CAD build for the part. Positions are in the model's coordinates, mm. A direction names the side the tool comes from. Coordinates: 2 decimals unless noted, no trailing zeros. Order: outer loops, then holes, each group sorted by start corner. A loop starts at its lowest first (then second) coordinate and runs counter-clockwise, first axis right, second up. Notation, with made-up numbers: M 84.25,70 L 104.25,70 A32 ccw 104.25,109 Z; hole C -13,41.25 d7. An arc over 180 degrees is marked long. One line per item, written item: value.
from build123d import *

# Parameters (mm, degrees)
SKETCH1_W           = 138
SKETCH1_H           = 95
BOSS_EXTRUDE1_DEPTH = 15
SKETCH2_W           = 128
SKETCH2_H           = 86
CUT_EXTRUDE1_DEPTH  = 7
SNAP_START          = 64.5
SNAP_HOOK2_DEPTH    = 2
SNAP_HOOK2_2_DEPTH  = 2
FILLET1_R           = 1
FILLET2_R           = 0.5
BOSS_EXTRUDE2_DEPTH = 2
FILLET3_R           = 0.5
FILLET4_R           = 0.5
FILLET7_R           = 0.1


with BuildPart() as part:
    # Sketch1 → Boss-Extrude1 (new body)
    with BuildSketch(Plane(origin=(0, 0, 0), x_dir=(1, 0, 0), z_dir=(0, 1, 0))):
        Rectangle(SKETCH1_W, SKETCH1_H)
    extrude(amount=BOSS_EXTRUDE1_DEPTH)

    # Sketch2 → Cut-Extrude1 (cut)
    with BuildSketch(Plane(origin=(0, 15, 0), x_dir=(1, 0, 0), z_dir=(0, 1, 0))):
        Rectangle(SKETCH2_W, SKETCH2_H)
    extrude(amount=-CUT_EXTRUDE1_DEPTH, mode=Mode.SUBTRACT)



with BuildPart() as body_2:
    # Snap Hook2: read off the stored shape, not the designer's step
    # Snap Hook2 outline → Snap Hook2 (new body)
    with BuildSketch(Plane.YZ.offset(SNAP_START)):
        Polygon((21, -2), (21, 2), (18, 2.157223338), (18, -2.157223338), align=None)
    snap_hook2 = extrude(amount=SNAP_HOOK2_DEPTH)


with BuildPart() as part_1:
    add(part.part)

    add(body_2.part)  # Snap Hook2 2 merges body 2
    # Snap Hook2 2 outline → Snap Hook2 2 (add)
    with BuildSketch(Plane.YZ.offset(SNAP_START)):
        Polygon((18, -2.157223338), (18, 2.157223338), (15, 2.314446676), (15, -2.314446676), align=None)
    snap_hook2_2 = extrude(amount=SNAP_HOOK2_2_DEPTH)

    # Snap Hook2 3: loft between two sections, ruled curve by curve
    snap_hook2_3_from = [
        Edge.make_line((66.5, 21, -2), (66.5, 21, 2)),
        Edge.make_line((66.5, 18, 2.157223338), (66.5, 18, -2.157223338)),
        Edge.make_line((66.5, 18, 2.157223338), (66.5, 21, 2)),
        Edge.make_line((66.5, 18, -2.157223338), (66.5, 21, -2)),
    ]
    snap_hook2_3_to = [
        Edge.make_line((68.5, 19, -2.104815559), (68.5, 19, 2.104815559)),
        Edge.make_line((68.5, 18, 2.157223338), (68.5, 18, -2.157223338)),
        Edge.make_line((68.5, 18, 2.157223338), (68.5, 19, 2.104815559)),
        Edge.make_line((68.5, 18, -2.157223338), (68.5, 19, -2.104815559)),
    ]
    snap_hook2_3 = Solid(Shell([*[Face.make_surface_from_curves(snap_hook2_3_from[k], snap_hook2_3_to[k]) for k in range(4)], Face(Wire(snap_hook2_3_from)), Face(Wire(snap_hook2_3_to))]))
    add(snap_hook2_3)

    # Fillet1
    fillet1_edges = [part_1.edges().sort_by_distance(p)[0] for p in [
        (64, 11.5, -43),
        (64, 11.5, 43),
        (-64, 11.5, 43),
        (-64, 11.5, -43),
        (-69, 7.5, -47.5),
        (69, 7.5, -47.5),
        (69, 7.5, 47.5),
        (-69, 7.5, 47.5),
    ]]
    fillet(fillet1_edges, radius=FILLET1_R)

    # Mirror1: Snap Hook2, Snap Hook2 2, Snap Hook2 3 across plane
    add(snap_hook2.mirror(Plane(origin=(0, 0, 0), x_dir=(0, 0, 1), z_dir=(1, 0, 0))))
    add(snap_hook2_2.mirror(Plane(origin=(0, 0, 0), x_dir=(0, 0, 1), z_dir=(1, 0, 0))))
    add(snap_hook2_3.mirror(Plane(origin=(0, 0, 0), x_dir=(0, 0, 1), z_dir=(1, 0, 0))))

    # Fillet2
    fillet2_edges = [part_1.edges().sort_by_distance(p)[0] for p in [
        (66.5, 15, 0),
        (64.5, 15, 0),
        (-66.5, 15, 0),
        (-64.5, 15, 0),
    ]]
    fillet(fillet2_edges, radius=FILLET2_R - 0.0001)  # a hair under: the kernel refuses the full size

    # Sketch5 → Boss-Extrude2 (add)
    with BuildSketch(Plane.ZY.offset(68.5)):
        Polygon((-2.104815559, 19), (2.104815559, 19), (2.189499682, 17.384130663), (-2.189499682, 17.384130663), align=None)
    extrude(amount=BOSS_EXTRUDE2_DEPTH)

    # Cut-Sweep1: sweep along a curve in space
    with BuildLine() as cut_sweep1_path:
        Line((-70.5, 17.384130663, -2.189499682), (-70.5, 17.384130663, 2.189499682))
    # Sketch6 → Cut-Sweep1 (sweep, cut)
    with BuildSketch(Plane(origin=(0, 0.162048562, -3.09207076), x_dir=(-1, 0, 0), z_dir=(0, 0.052335956242943814, -0.998629534754574))):
        Polygon((68.5, 17.862431279), (69.245478091, 17.245716756), (68.5, 17.245716756), align=None)
    sweep(path=cut_sweep1_path.line, mode=Mode.SUBTRACT)

    # Cut-Sweep2: sweep along a curve in space
    with BuildLine() as cut_sweep2_path:
        Line((-70.5, 17.384130663, -2.189499682), (-70.5, 17.384130663, 2.189499682))
    # Sketch7 → Cut-Sweep2 (sweep, cut)
    with BuildSketch(Plane(origin=(0, 0.162048562, -3.09207076), x_dir=(-1, 0, 0), z_dir=(0, 0.052335956242943814, -0.998629534754574))):
        Polygon((68.5, 18.863803625), (69.5, 17.245716756), (70.5, 17.245716756), (70.5, 18.863803625), align=None)
    sweep(path=cut_sweep2_path.line, mode=Mode.SUBTRACT)

    # Fillet3
    # the kernel refuses this fillet: 0.5 mm, written as the material it adds along each edge
    with BuildSketch(Plane(origin=(-68.5, 18, 2.606776404), x_dir=(1, 0, 0), z_dir=(0, 0, -1))) as fillet3_piece_1_section:
        with BuildLine():
            CenterArc((FILLET3_R * 0.359642452732, FILLET3_R), FILLET3_R, 230.43852258, 39.56147742)
            Line((-FILLET3_R * 0.277263341593, FILLET3_R * 0.22905836203), (0, 0))
            Line((0, 0), (FILLET3_R * 0.359642452732, 0))
        make_face()
    fillet3_piece_1 = extrude(amount=5.213552808, mode=Mode.PRIVATE)
    fillet3_piece_1 = split(fillet3_piece_1, bisect_by=Plane(origin=(-68.5, 17.976504454, 2.158454687), z_dir=(0, -0.052335956242943654, -0.9986295347545739)), keep=Keep.TOP, mode=Mode.PRIVATE)
    fillet3_piece_1 = split(fillet3_piece_1, bisect_by=Plane(origin=(-68.5, 18.248986786, -2.144174493), z_dir=(0, -0.05233595624294393, 0.9986295347545739)), keep=Keep.TOP, mode=Mode.PRIVATE)
    add(fillet3_piece_1)
    # the kernel refuses this fillet: 0.5 mm, written as the material it takes off along each edge
    with BuildSketch(Plane(origin=(-68.5, 19, -2.249978478), x_dir=(0.7071067811865781, 0.7071067811865169, 0), z_dir=(0, 0, 1))) as fillet3_2_piece_1:
        with BuildLine():
            CenterArc((FILLET3_R * 0.11613033532, -FILLET3_R), FILLET3_R, 90, 13.248212602)
            Line((-FILLET3_R * 0.11303968997, -FILLET3_R * 0.0266135918822), (0, 0))
            Line((0, 0), (FILLET3_R * 0.11613033532, 0))
        make_face()
    extrude(amount=4.499956956, mode=Mode.SUBTRACT)

    # Fillet4
    # the kernel refuses this fillet: 0.5 mm, written as the material it takes off along each edge
    with BuildSketch(Plane(origin=(-69.5, 17.384130663, -3.553874189), x_dir=(0.5262404509675064, 0.8503358088223238, 0), z_dir=(0, 0, 1))) as fillet4_piece_1:
        with BuildLine():
            CenterArc((0.545749803, -0.5), FILLET4_R, 90, 55.448844763)
            Line((0.133939724, -0.216429093), (0.125703523, -0.210757675))
            ThreePointArc((0.125703523, -0.210757675), (0.058466504, -0.113476951), (-0.008503358, -0.005262405))
            Line((-0.008503358, -0.005262405), (0, 0.01))
            Line((0, 0.01), (0.545749803, 0.01))
            Line((0.545749803, 0.01), (0.545749803, 0))
        make_face()
    extrude(amount=7.107748378, mode=Mode.SUBTRACT)

    # Fillet7
    fillet7_edges = [part_1.edges().sort_by_distance(p)[0] for p in [
        (-69.245478091, 17.384130663, 0),
    ]]
    fillet(fillet7_edges, radius=FILLET7_R)


solid = part_1.part
Q1. Slice it at A-A (x = 38). List the corners of the cut face in (y, z).
Recorded:
outline: M 0,-47.5 L 15,-47.5 L 15,-43 L 8,-43 L 8,43 L 15,43 L 15,47.5 L 0,47.5 Z
Q2. Mould opens along Z. For faces 1 (the face through (-65.48, 17.96, -2.16)), 2 (the face through (-1, 8, -1)), 3 (the face through (-1, 0, -1)) say: released by +Z, released by -Z, zero draft, split by the parting line, or undercut.
Recorded:
face 1: released by -Z
face 2: undercut
face 3: zero draft
Q3. Pin check, flat tips, straight feed: pin 1 Ø7.5 at (y, z) = (12.5, 20.5) entering from -X; pin 2 Ø6 at (x, z) = (-14, -14) entering from +Y; pin 3 Ø0.8 at (y, z) = (18.5, -0.5) entering from +X. Stop position of each tip, or through.
Recorded:
pin 1: stops at x = -69
pin 2: stops at y = 8
pin 3: stops at x = 68.5
Q4. Drill centre lines: line 1 along X through (y, z) = (14.25, -37); line 2 along X through (y, z) = (2.75, -13); line 3 along Y through (x, z) = (-27.5, 5). Where is each one in solid material? Low to high.
Recorded:
line 1: x = -69 to -64, 64 to 69
line 2: x = -69 to 69
line 3: y = 0 to 8
Q5. Slice it at B-B (z = -32.5). List the corners of the cut face in (x, y).
Recorded:
outline: M -69,0 L 69,0 L 69,15 L 64,15 L 64,8 L -64,8 L -64,15 L -69,15 Z
Q6. Which spindle directions (+Z, -Z, +X, -X, +Y, -Y) get a long thin tool onto all of the face, cutting with end or side? Do faces 4 (the face through (-64, 12, 1)), 5 (the face through (-64.5, 18, 0)), 6 (the face through (-65.812, 18.042, 2.155)). Say none if no direction does.
Recorded:
face 4: +Y
face 5: +Z, -Z, +Y
face 6: +Z, +X, -X, +Y
